Geometry: final body of the model. Coordinates: model frame, mm. Face numbers are marked on the shaded views. A direction names the side the tool comes from. Give positions to 0.01 mm unless a question says otherwise; leave off trailing zeros. Write each loop counter-clockwise with the first axis right and the second up, starting at its lowest first coordinate (ties: lowest second). Pieces come first, ordered by that corner, then holes. Notation, with made-up numbers: M -32.5,-12.5 L 8.5,-12.5 A20 cw 8.5,-6.5 Z; hole C 77,22.5 d11. An arc over 180 degrees is marked long. Use one line per item in the form item = value. Start each with the question number.
Item 1: Section query D-D on x = 35.75. Return loops of the section in (y, z), then the cut area to 3 significant figures.
Item 2: Pull-direction query (Y, two-part tool) for the marked faces 1, 2, 3 and 4; classes: released by +Y, released by -Y, zero draft, split by the parting line, or undercut.
Item 3: Section query C-C on y = -30. Return loops of the section in (x, z), then the cut area to 3 significant figures.
Item 4: Access query for the marked faces 5 and 6. Directions: +Z, -Z, +X, -X, +Y, -Y. A direction counts if a zero-diameter tool reaches every point of the face in a straight line with its end or side. Return the directions, or none.
Item 5: Contact query for flat-ended pins moving along their axis: P1, Ø2, axis at x = 35.5, y = -31, coming from the +Z side; P2, Ø1.5, axis at x = 37, y = -31, coming from the -Z side. Output: stop coordinate, or through.
Item 6: Section query A-A on x = 37.75. Return loops of the section in (y, z), then the cut area to 3 significant figures.
Item 7: Section query B-B on z = 7.75. Return loops of the section in (x, y).
Item 8: Material intervals for line 1 along Y through (x, z) = (33, 3.5); line 2 along X through (y, z) = (-27.75, 4.5); line 3 along Z through (x, y) = (32.5, -21), sorted ascending. Write a range as from..to.
from build123d import *

# Parameters (mm, degrees)
F0_W     = 14
F0_H     = 17
F1_DEPTH = 1
F2_W     = 14
F2_H     = 17
F2_W_2   = 12
F2_H_2   = 15
F3_DEPTH = 7
F5_D     = 1


with BuildPart() as f1:
    # F0 (on Top) → F1 (new body)
    with BuildSketch(Plane.XY):
        with Locations((33.291668, -25.269144)):
            Rectangle(F0_W, F0_H)
    extrude(amount=F1_DEPTH)

    # F2 (on face) → F3 (join)
    with BuildSketch(Plane.XY.offset(1)):
        with Locations((33.291668, -25.269144)):
            Rectangle(F2_W, F2_H)
        with Locations((33.291668, -25.269144)):
            Rectangle(F2_W_2, F2_H_2, mode=Mode.SUBTRACT)
    extrude(amount=F3_DEPTH)

    # F5 (through all)
    with Locations(Plane.XY.offset(1)):
        with Locations((28.405087, -31.885728), (37.959054, -31.737298)):
            Hole(F5_D / 2)


solid = f1.part
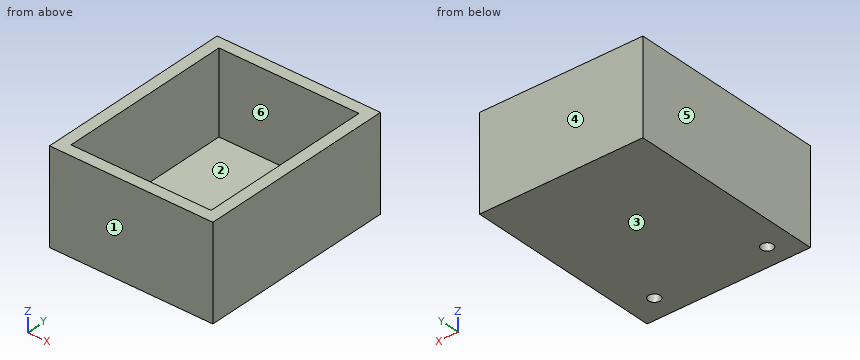
Answer sheet:
q1.outline = M -33.77,0 L -16.77,0 L -16.77,8 L -17.77,8 L -17.77,1 L -32.77,1 L -32.77,8 L -33.77,8 Z
q1.area = 31.0 mm2
q2.face_1 = released by -Y
q2.face_2 = undercut
q2.face_3 = zero draft
q2.face_4 = released by +Y
q3.outline = M 26.29,0 L 40.29,0 L 40.29,8 L 39.29,8 L 39.29,1 L 27.29,1 L 27.29,8 L 26.29,8 Z
q3.area = 28.0 mm2
q4.face_5 = +Z, -Z, -X, +Y, -Y
q4.face_6 = +Z
q5.P1 = 1
q5.P2 = 0
q6.outline = M -33.77,0 L -32.19,0 L -32.19,1 L -32.77,1 L -32.77,8 L -33.77,8 Z; M -31.28,0 L -16.77,0 L -16.77,8 L -17.77,8 L -17.77,1 L -31.28,1 Z
q6.area = 30.1 mm2
q7.outline = M 26.29,-33.77 L 40.29,-33.77 L 40.29,-16.77 L 26.29,-16.77 Z; hole M 27.29,-32.77 L 39.29,-32.77 L 39.29,-17.77 L 27.29,-17.77 Z
q8.line_1 = -33.77..-32.77, -17.77..-16.77
q8.line_2 = 26.29..27.29, 39.29..40.29
q8.line_3 = 0..1
